```python
from build123d import *

# Parameters (mm, degrees)
SKETCH_1_W             = 62.2
SKETCH_1_H             = 62.2
EXTRUDE_1_DEPTH        = 37
SKETCH_2_R             = 15
EXTRUDE_2_DEPTH        = 5
SKETCH_3_R             = 13.5
EXTRUDE_3_DEPTH        = 5
SKETCH_4_R             = 15
EXTRUDE_4_DEPTH        = 5
SKETCH_5_R             = 14
EXTRUDE_5_DEPTH        = 20
SKETCH_6_R             = 26
EXTRUDE_6_DEPTH        = 70
SKETCH_7_R             = 27
EXTRUDE_7_DEPTH        = 5
SKETCH_8_R             = 14.5
CUT_EXTRUDE_1_DEPTH    = 0.5
SKETCH_9_R             = 4.987570285
SKETCH_9_R_2           = 3.46960963
EXTRUDE_8_DEPTH        = 7
SKETCH_10_W            = 8.223130645
SKETCH_10_H            = 5.124180357
CUT_EXTRUDE_2_DEPTH    = 3
HOLE_WIZARD_M4_1_D     = 3.3
HOLE_WIZARD_M4_1_DEPTH = 10.1
HOLE_WIZARD_M4_1_TIP   = 0.991420021
HOLE_WIZARD_M4_2_D     = 3.3
HOLE_WIZARD_M4_2_DEPTH = 10.1
HOLE_WIZARD_M4_2_TIP   = 0.991420021
HOLE_WIZARD_M4_3_D     = 3.3
HOLE_WIZARD_M4_3_DEPTH = 10.1
HOLE_WIZARD_M4_3_TIP   = 0.991420021
HOLE_WIZARD_M4_4_D     = 3.3
HOLE_WIZARD_M4_4_DEPTH = 10.1
HOLE_WIZARD_M4_4_TIP   = 0.991420021


with BuildPart() as part:
    # 草图1 → 凸台-拉伸1 (new body)
    with BuildSketch(Plane.XY):
        with Locations((31.1, 31.1)):
            Rectangle(SKETCH_1_W, SKETCH_1_H)
    extrude(amount=EXTRUDE_1_DEPTH)

    # 草图2 → 凸台-拉伸2 (add)
    with BuildSketch(Plane.XY.offset(37)):
        with Locations(Location((31.1, 31.1, 0), (0, 0, 180))):
            Circle(SKETCH_2_R)
    extrude(amount=EXTRUDE_2_DEPTH)

    # 草图3 → 凸台-拉伸3 (add)
    with BuildSketch(Plane.XY.offset(42)):
        with Locations((31.1, 31.1)):
            Circle(SKETCH_3_R)
    extrude(amount=EXTRUDE_3_DEPTH)

    # 草图4 → 凸台-拉伸4 (add)
    with BuildSketch(Plane.XY.offset(47)):
        with Locations(Location((31.1, 31.1, 0), (0, 0, 180))):
            Circle(SKETCH_4_R)
    extrude(amount=EXTRUDE_4_DEPTH)

    # 草图5 → 凸台-拉伸5 (add)
    with BuildSketch(Plane.XY.offset(52)):
        with Locations((31.1, 31.1)):
            Circle(SKETCH_5_R)
    extrude(amount=EXTRUDE_5_DEPTH)

    # 草图6 → 凸台-拉伸6 (add)
    with BuildSketch(Plane.XY.offset(72)):
        with Locations((31.1, 31.1)):
            Circle(SKETCH_6_R)
    extrude(amount=EXTRUDE_6_DEPTH)

    # 草图7 → 凸台-拉伸7 (add)
    with BuildSketch(Plane.XY.offset(142)):
        with Locations((31.1, 31.1)):
            Circle(SKETCH_7_R)
    extrude(amount=EXTRUDE_7_DEPTH)

    # 草图8 → 切除-拉伸1 (cut)
    with BuildSketch(Plane.XY.offset(147)):
        with Locations((31.1, 31.1)):
            Circle(SKETCH_8_R)
    extrude(amount=-CUT_EXTRUDE_1_DEPTH, mode=Mode.SUBTRACT)

    # 草图9 → 凸台-拉伸8 (add)
    with BuildSketch(Plane(origin=(0, 0, 0), x_dir=(-1, 0, 0), z_dir=(0, 0, -1))):
        with Locations((-16.576254003, 47.30330958)):
            Circle(SKETCH_9_R)
        with Locations((-16.576254003, 47.30330958)):
            Circle(SKETCH_9_R_2, mode=Mode.SUBTRACT)
    extrude(amount=EXTRUDE_8_DEPTH)

    # 草图10 → 切除-拉伸2 (cut)
    with BuildSketch(Plane(origin=(0, 0, 0), x_dir=(-1, 0, 0), z_dir=(0, 0, -1))):
        with Locations((-20.516916702, 15.688590304)):
            Rectangle(SKETCH_10_W, SKETCH_10_H)
    extrude(amount=-CUT_EXTRUDE_2_DEPTH, mode=Mode.SUBTRACT)

    # M4 螺纹孔1
    with Locations(Plane(origin=(0, 62.2, 0), x_dir=(-1, 0, 0), z_dir=(0, 1, 0))):
        with Locations((-10.1, 32.5), (-52.1, 32.5)):
            Hole(HOLE_WIZARD_M4_1_D / 2, depth=HOLE_WIZARD_M4_1_DEPTH)
            with Locations((0, 0, -(HOLE_WIZARD_M4_1_DEPTH + HOLE_WIZARD_M4_1_TIP / 2))):  # 118° drill point
                Cone(0, HOLE_WIZARD_M4_1_D / 2, HOLE_WIZARD_M4_1_TIP, mode=Mode.SUBTRACT)

    # M4 螺纹孔2
    with Locations(Plane(origin=(62.2, 0, 0), x_dir=(0, 0, -1), z_dir=(1, 0, 0))):
        with Locations((-32.5, 10.1), (-32.5, 52.1)):
            Hole(HOLE_WIZARD_M4_2_D / 2, depth=HOLE_WIZARD_M4_2_DEPTH)
            with Locations((0, 0, -(HOLE_WIZARD_M4_2_DEPTH + HOLE_WIZARD_M4_2_TIP / 2))):  # 118° drill point
                Cone(0, HOLE_WIZARD_M4_2_D / 2, HOLE_WIZARD_M4_2_TIP, mode=Mode.SUBTRACT)

    # M4 螺纹孔3
    with Locations(Plane.XZ):
        with Locations((10.1, 32.5), (52.1, 32.5)):
            Hole(HOLE_WIZARD_M4_3_D / 2, depth=HOLE_WIZARD_M4_3_DEPTH)
            with Locations((0, 0, -(HOLE_WIZARD_M4_3_DEPTH + HOLE_WIZARD_M4_3_TIP / 2))):  # 118° drill point
                Cone(0, HOLE_WIZARD_M4_3_D / 2, HOLE_WIZARD_M4_3_TIP, mode=Mode.SUBTRACT)

    # M4 螺纹孔4
    with Locations(Plane.ZY):
        with Locations((32.5, 52.1), (32.5, 10.1)):
            Hole(HOLE_WIZARD_M4_4_D / 2, depth=HOLE_WIZARD_M4_4_DEPTH)
            with Locations((0, 0, -(HOLE_WIZARD_M4_4_DEPTH + HOLE_WIZARD_M4_4_TIP / 2))):  # 118° drill point
                Cone(0, HOLE_WIZARD_M4_4_D / 2, HOLE_WIZARD_M4_4_TIP, mode=Mode.SUBTRACT)


solid = part.part
```
Model file for the job. Use its own axes, mm. A direction names the side the tool comes from. Give positions to 0.01 mm unless a question says otherwise; leave off trailing zeros. Loops run counter-clockwise (first coordinate to the right, second up) from the corner with the lowest first, then second, coordinate; pieces in that order, holes last. Notation, with made-up numbers: (50.25, -24.75) -> (81.25, -24.75) arc R24 cw to (81.25, 5.25) -> close; hole circle Ø1 at (-34, -12). An arc over 180 degrees is marked (long way). Use CSV: the item, a comma, the result in double quotes. Start each with the question number.
1) Wall check: line 1 (Z direction, x = 10.1, y = 54.5); line 2 (Z direction, x = 48.5, y = 31.5); line 3 (Z direction, x = 29, y = 25). Give the ranges that are in metal, low to high.
2) Tool access for faces 1 (the flat face through (24.628, 16, 1)), 2 (the cylindrical face through (5.1, 50.5, 32.9)), 3 (the flat face through (42, 20, 72)), 4 (the cylindrical face through (57.079, 11.736, 32.285)): list every direction of +Z, -Z, +X, -X, +Y, -Y with a clear straight run to the whole face (end or side of a thin tool).
3) Mould opens along X. For faces 5 (the flat face through (20, 46, -7)), 6 (the cylindrical face through (33.053, 16.228, 49.465)), 7 (the flat face through (16.405, 16, 1)) say: released by +X, released by -X, zero draft, split by the parting line, or undercut.
4) Flat gauge pins, fed straight in: pin 1 Ø1.5 at (x, y) = (16, 55) entering from +Z; pin 2 Ø4 at (x, y) = (22, 15.5) entering from -Z; pin 3 Ø24 at (x, y) = (31, 37.5) entering from -Z. Where does each tip first touch, or does it go through?
5) Slice it at C-C on z = 122. Give the cut face in (x, y).
Computed values:
1,line 1,"z = 0 to 30.85, 34.15 to 37"
1,line 2,"z = 0 to 37, 72 to 147"
1,line 3,"z = 0 to 146.5"
2,face 1,"-Z"
2,face 2,"-X"
2,face 3,"none"
2,face 4,"+X"
3,face 5,"zero draft"
3,face 6,"split by the parting line"
3,face 7,"undercut"
4,pin 1,"stops at z = 37"
4,pin 2,"stops at z = 3"
4,pin 3,"stops at z = 0"
5,outline,"circle Ø52 at (31.1, 31.1)"
